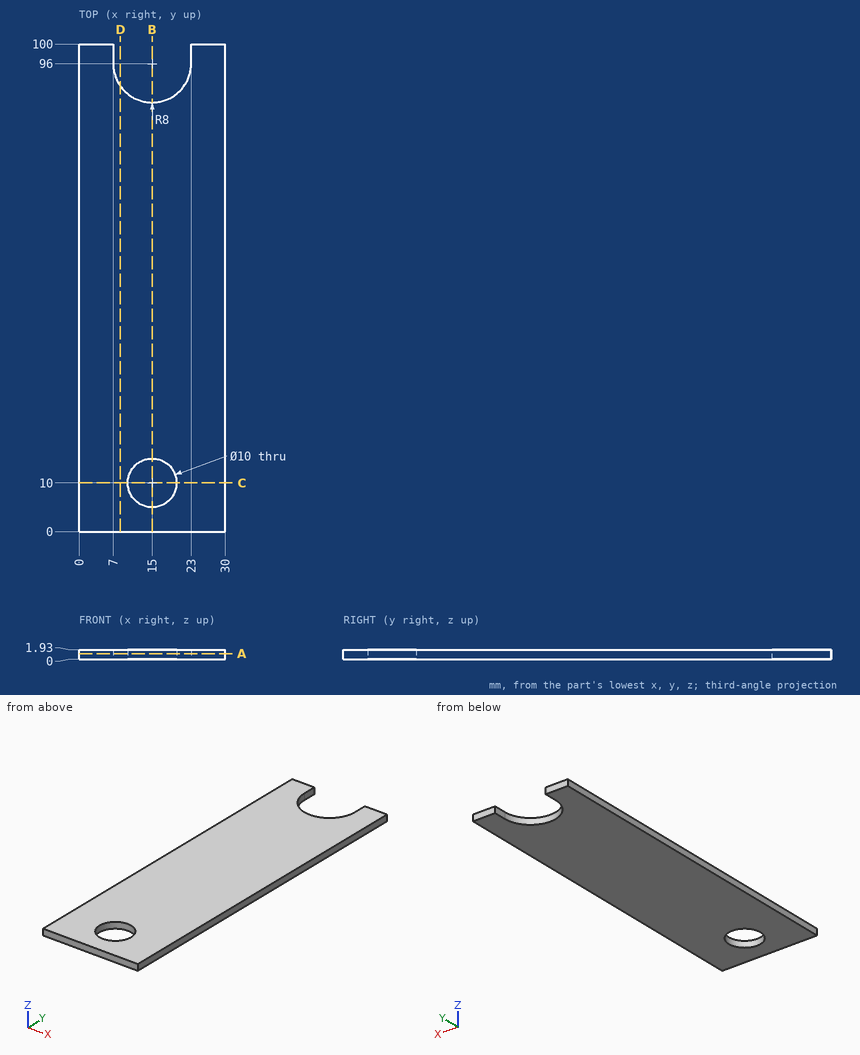
Geometry check sheet. Reference: drawing and pictorial views, mm from the part's lowest x, y, z. Round coordinates to 2 decimals unless told otherwise and drop trailing zeros. Loops run counter-clockwise (first coordinate to the right, second up) from the corner with the lowest first, then second, coordinate; pieces in that order, holes last. Notation, with made-up numbers: (62, 7) - (75, 7) arc R10 ccw to (75, 15) - close; hole circle Ø6 at (72.25, 28). An arc over 180 degrees is marked (long way). Answer in a Markdown table with one row per item. Add a question column.
Q1. Gauge pin test, flat ends, axial feed: pin 1 (12 mm diameter, centred on x = 6.5, y = 52.5, fed in from -Z); pin 2 (9 mm diameter, centred on x = 15, y = 10, fed in from -Z). Record the tip position at first contact, or that the pin passes through.
Q2. Section check C-C on y = 10. Enter the section's corners in (x, z).
Q3. Section check A-A on z = 1.1. Enter the section's corners in (x, y).
Q4. Section check B-B on x = 15. Enter the section's corners in (y, z), plus the area to 3 significant figures.
Q5. Material ranges on line 1 (Y direction, x = 15, z = 0.4); line 2 (Y direction, x = 12.5, z = 1.45); line 3 (X direction, y = 10.5, z = 0.5), recorded low to high.
Q6. Section check D-D on x = 8.5. Enter the section's corners in (y, z).
Found:
| question | item | result |
|---|---|---|
| 1 | pin 1 | stops at z = 0 |
| 1 | pin 2 | passes through |
| 2 | outline | (0, 0) - (10, 0) - (10, 1.93) - (0, 1.93) - close; (20, 0) - (30, 0) - (30, 1.93) - (20, 1.93) - close |
| 3 | outline | (0, 0) - (30, 0) - (30, 100) - (23, 100) - (23, 96) arc R8 cw to (7, 96) - (7, 100) - (0, 100) - close; hole circle Ø10 at (15, 10) |
| 4 | outline | (0, 0) - (5, 0) - (5, 1.93) - (0, 1.93) - close; (15, 0) - (88, 0) - (88, 1.93) - (15, 1.93) - close |
| 4 | area | 151 mm² |
| 5 | line 1 | y = 0 to 5, 15 to 88 |
| 5 | line 2 | y = 0 to 5.67, 14.33 to 88.4 |
| 5 | line 3 | x = 0 to 10.03, 19.97 to 30 |
| 6 | outline | (0, 0) - (91.34, 0) - (91.34, 1.93) - (0, 1.93) - close |
